```python
from build123d import *

# Parameters (mm, degrees)
CYLINDER_R     = 1.4
CYLINDER_DEPTH = 10
ARRAY001_COUNT = 3
SKETCH018_W    = 3.15
SKETCH018_H    = 2.3
SKETCH002_W    = 5
SKETCH002_H    = 6.8
ARRAY_Z_COUNT  = 6
ARRAY_Z_PITCH  = 1.6


with BuildPart() as boltholes:
    # Cylinder → Cylinder (new body)
    with BuildSketch(Plane(origin=(0, 6, -1), x_dir=(1, 0, 0), z_dir=(0, 0, 1))):
        Circle(CYLINDER_R)
    extrude(amount=CYLINDER_DEPTH)

    # Array001: BoltHoles ×3 about axis
    array001_axis = Axis((0, 0, 0), (0, 0, 1))


with BuildPart() as boltholes_1:
    add(boltholes.part)
    for i in range(1, ARRAY001_COUNT):
        add(boltholes.part.rotate(array001_axis, i * 360 / ARRAY001_COUNT))


with BuildPart() as obj1:
    # Sketch018 → Revolution007 (revolve)
    with BuildSketch(Plane.XZ):
        with Locations((1.575, 5.7267413876)):
            Rectangle(SKETCH018_W, SKETCH018_H)
    revolve(axis=Axis((0, 0, 0), (0, 0, 1)))


with BuildPart() as obj2:
    # Sketch007 → Revolution006 (revolve)
    with BuildSketch(Plane.XZ):
        with BuildLine():
            ThreePointArc((1.5, 1.7955317108), (0.867020761, 2.4322916436), (0, 2.6655317108))
            Line((0, 2.6655317108), (0, 0.7955317108))
            Line((0, 0.7955317108), (1.5, 0.7955317108))
            Line((1.5, 1.7955317108), (1.5, 0.7955317108))
        make_face()
    revolve(axis=Axis((0, 0, 0), (0, 0, 1)))


with BuildPart() as obj3:
    # Sketch002 → Revolution002 (revolve)
    with BuildSketch(Plane.XZ):
        with Locations((7.5, 3.8)):
            Rectangle(SKETCH002_W, SKETCH002_H)
    revolve(axis=Axis((0, 0, 0), (0, 0, 1)))


with BuildPart() as innergroovetool:
    # Sketch001 → Revolution001 (revolve)
    with BuildSketch(Plane.XZ):
        Polygon((4, 8), (4, 6.4), (8, 6.4), (8.8, 7.2), (8, 8), align=None)
    revolve(axis=Axis((0, 0, 0), (0, 0, 1)))

    # Array Z: InnerGrooveTool ×6


with BuildPart() as innergroovetool_1:
    add(innergroovetool.part)
    with Locations(*[(0, 0, -i * ARRAY_Z_PITCH) for i in range(1, ARRAY_Z_COUNT)]):
        add(innergroovetool.part)

    # Common: intersect obj3
    add(obj3.part, mode=Mode.INTERSECT)


with BuildPart() as boltholes001:
    # Sketch → Revolution (revolve)
    with BuildSketch(Plane.XZ):
        Polygon((1.2, 0.4), (8, 0.4), (8, 7.2), (2.8, 7.2), (1.2, 2.2), align=None)
    revolve(axis=Axis((0, 0, 0), (0, 0, 1)))

    # Fusion001: union InnerGrooveTool
    add(innergroovetool_1.part)

    # Cut: cut obj2
    add(obj2.part, mode=Mode.SUBTRACT)

    # Cut003: cut obj1
    add(obj1.part, mode=Mode.SUBTRACT)

    # Cut001: cut BoltHoles
    add(boltholes_1.part, mode=Mode.SUBTRACT)


solid = boltholes001.part
```
Model file for the job. Use its own axes, mm. Round coordinates to 2 decimals unless told otherwise and drop trailing zeros. Write each loop counter-clockwise with the first axis right and the second up, starting at its lowest first coordinate (ties: lowest second). Pieces come first, ordered by that corner, then holes. Notation, with made-up numbers: (-6.5, 26.25) - (51.5, 26.25) arc R15 ccw to (51.5, 33.25) - close; hole circle Ø1 at (67.25, -17). An arc over 180 degrees is marked (long way). Use CSV: the item, a comma, the result in double quotes. Start each with the question number.
Item 1: Drill centre lines: L1, parallel to Z at x = -2, y = -8; L2, parallel to Y at x = 0, z = 0.5; L3, parallel to Z at x = -5, y = 7. Where is each one in solid material? Low to high. Write a range as [from, to].
Item 2: Pin check, flat tips, straight feed: P1, Ø4.5, axis at x = 5.2, y = -3, coming from the -Z side; P2, Ø2, axis at y = 1, z = 5.5, coming from the +X side. Stop position of each tip, or through.
Item 3: Two-plate mould, pull along Z, no slides. Class faces 1 (the face through (2.1, 2.1, 7.2)), 2 (the face through (-4.55, -4.24, 3.75)), 3 (the face through (-2, -1, 4.577)): released by +Z, released by -Z, zero draft, split by the parting line, or undercut.
Item 4: Band-saw the part on A-A (z = 5.25). Write the cut outline in (x, y), and give its area (3 significant figures).
Item 5: Band-saw the part on B-B (x = 0). State how many separate pieces and enclosed holes the cut face has, and give its area (3 significant figures).
Checked values:
1,L1,"z = [0.4, 1.35], [1.85, 2.95], [3.45, 4.55], [5.05, 6.15], [6.65, 7.2]"
1,L2,"y = [-8.5, -1.2], [1.2, 4.6], [7.4, 8.5]"
1,L3,"z = [0.6, 1], [2.2, 2.6], [3.8, 4.2], [5.4, 5.8], [7, 7.2]"
2,P1,"stops at z = 0.4"
2,P2,"stops at x = 8.8"
3,face 1,"released by +Z"
3,face 2,"zero draft"
3,face 3,"undercut"
4,outline,"circle Ø16.9 at (0, 0); hole circle Ø2.8 at (-5.2, -3); hole circle Ø6.3 at (0, 0); hole circle Ø2.8 at (0, 6); hole circle Ø2.8 at (5.2, -3)"
4,area,"175 mm²"
5,separate pieces,"3"
5,enclosed holes,"0"
5,area,"66.5 mm²"
